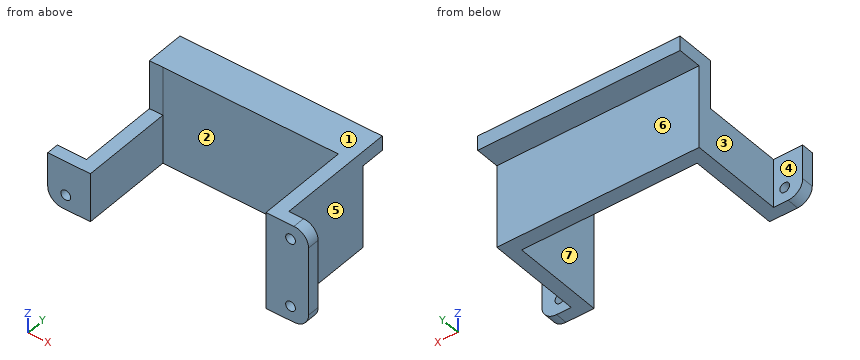
from build123d import *

# Parameters (mm, degrees)
BOSS_EXTRUDE1_DEPTH      = 33.5
SKETCH2_W                = 20
SKETCH2_H                = 2.5
BOSS_EXTRUDE2_DEPTH      = 6
SKETCH9_R                = 1
CORTE_EXTRUS_O1_DEPTH    = 48.67140128
FILETE1_R                = 3
ESBO_O12_W               = 41.5
ESBO_O12_H               = 3
RESSALTO_EXTRUS_O1_DEPTH = 5
FILETE1_OF_ESPELHAR1_R   = 3
ESBO_O14_W               = 12
ESBO_O14_H               = 19.002666305
CORTE_EXTRUS_O10_DEPTH   = 10
ESBO_O15_W               = 13.5
ESBO_O15_H               = 22.081303671
CORTE_EXTRUS_O11_DEPTH   = 62.469504634


with BuildPart() as part:
    # Sketch1 → Boss-Extrude1 (new body)
    with BuildSketch(Plane.XY):
        Polygon((19, -20), (21.75, -20), (21.75, 2), (-19.75, 2), (-19.75, -20), (-17, -20), (-17, -1), (19, -1), align=None)
    extrude(amount=BOSS_EXTRUDE1_DEPTH)

    # Sketch2 → Boss-Extrude2 (add)
    with BuildSketch(Plane(origin=(21.75, 0, 0), x_dir=(0, 0, -1), z_dir=(1, 0, 0))):
        with Locations((-23.5, -18.75)):
            Rectangle(SKETCH2_W, SKETCH2_H)
    boss_extrude2 = extrude(amount=BOSS_EXTRUDE2_DEPTH)

    # Sketch9 → Corte-extrusão1 (cut, through all)
    with BuildSketch(Plane(origin=(0, -17.5, 0), x_dir=(1, 0, 0), z_dir=(0, 1, 0))):
        with Locations(Location((24.05, -16.5, 0), (0, 0, 270))):
            Circle(SKETCH9_R)
        with Locations(Location((24.05, -30.5, 0), (0, 0, 270))):
            Circle(SKETCH9_R)
    corte_extrus_o1 = extrude(amount=-CORTE_EXTRUS_O1_DEPTH, mode=Mode.SUBTRACT)

    # Filete1
    filete1_edges = [part.edges().sort_by_distance(p)[0] for p in [
        (27.75, -18.75, 13.5),
        (27.75, -18.75, 33.5),
    ]]
    fillet(filete1_edges, radius=FILETE1_R)

    # Esboço12 → Ressalto-extrusão1 (add)
    with BuildSketch(Plane(origin=(0, 2, 0), x_dir=(1, 0, 0), z_dir=(0, 1, 0))):
        with Locations((1, -32)):
            Rectangle(ESBO_O12_W, ESBO_O12_H)
    extrude(amount=RESSALTO_EXTRUS_O1_DEPTH)

    # Espelhar1: Boss-Extrude2, Corte-extrusão1 across plane
    add(boss_extrude2.mirror(Plane(origin=(1, 0, 0), x_dir=(0, 0, 1), z_dir=(1, 0, 0))))
    add(corte_extrus_o1.mirror(Plane(origin=(1, 0, 0), x_dir=(0, 0, 1), z_dir=(1, 0, 0))), mode=Mode.SUBTRACT)

    # Filete1 of Espelhar1
    filete1_of_espelhar1_edges = [part.edges().sort_by_distance(p)[0] for p in [
        (-25.75, -18.75, 13.5),
        (-25.75, -18.75, 33.5),
    ]]
    fillet(filete1_of_espelhar1_edges, radius=FILETE1_OF_ESPELHAR1_R)

    # Esboço14 → Corte-extrusão10 (cut)
    with BuildSketch(Plane.XY.offset(33.5)):
        with Locations((-23, -10.498666848)):
            Rectangle(ESBO_O14_W, ESBO_O14_H)
    extrude(amount=-CORTE_EXTRUS_O10_DEPTH, mode=Mode.SUBTRACT)

    # Esboço15 → Corte-extrusão11 (cut, through all)
    with BuildSketch(Plane.ZY.offset(19.75)):
        with Locations((6.75, -8.959348164)):
            Rectangle(ESBO_O15_W, ESBO_O15_H)
    extrude(amount=-CORTE_EXTRUS_O11_DEPTH, mode=Mode.SUBTRACT)


solid = part.part
Check sheet for the modelled part. Datum: model origin and axes. Units: mm. Face numbers are marked on the shaded views. A direction names the side the tool comes from. Give positions to 0.01 mm unless a question says otherwise; leave off trailing zeros. Loops run counter-clockwise (first coordinate to the right, second up) from the corner with the lowest first, then second, coordinate; pieces in that order, holes last. Notation, with made-up numbers: M -10,-13 L 12,-13 A25 cw 12,6 Z; hole C 73,31.5 d6. An arc over 180 degrees is marked long. Answer as a JSON object with one key per item and string values. Group by question number.
Q1. Cross-section at C-C on x = 24.05. Record the cut outline in (y, z).
Q2. Cross-section at A-A on y = -13. Record the cut outline in (x, z).
Q3. Go/stop test with flat-tipped pins: P1, Ø5, axis at x = -23.5, z = 16, coming from the +Y side; P2, Ø6, axis at y = -12, z = 28.5, coming from the +X side; P3, Ø3, axis at x = -18, z = 29, coming from the -Y side. Record where each tip stops, or that it passes through.
Q4. Release check for a two-part mould opening along X. For the marked faces 1, 2 and 3 record: released by +X, released by -X, zero draft, split by the parting line, or undercut.
Q5. Material ranges on line 1 along X through (y, z) = (-18.4, 16.5); line 2 along X through (y, z) = (-16.5, 18); line 3 along Z through (x, y) = (-22.05, -19.5), recorded low to high. Write a range as [from, to].
Q6. Cross-section at B-B on x = -22.05. Record the cut outline in (y, z).
Q7. Access from +Z, -Z, +X, -X, +Y, -Y to the whole of each face (thin tool, end or side, straight path). Record for the marked faces 4, 5, 6 and 7.
Evaluation:
{
 "1": {"outline": "M -20,13.5 L -17.5,13.5 L -17.5,15.5 L -20,15.5 Z; M -20,17.5 L -17.5,17.5 L -17.5,29.5 L -20,29.5 Z; M -20,31.5 L -17.5,31.5 L -17.5,33.5 L -20,33.5 Z"},
 "2": {"outline": "M -19.75,13.5 L -17,13.5 L -17,23.5 L -19.75,23.5 Z; M 19,13.5 L 21.75,13.5 L 21.75,33.5 L 19,33.5 Z"},
 "3": {"P1": "stops at y = -17.5", "P2": "stops at x = 21.75", "P3": "stops at y = -1"},
 "4": {"face 1": "zero draft", "face 2": "undercut", "face 3": "released by -X"},
 "5": {"line 1": "x = [-25.75, -23.05], [-21.05, -17], [19, 23.05], [25.05, 27.75]", "line 2": "x = [-19.75, -17], [19, 21.75]", "line 3": "z = [13.5, 15.5], [17.5, 23.5]"},
 "6": {"outline": "M -20,13.5 L -17.5,13.5 L -17.5,15.5 L -20,15.5 Z; M -20,17.5 L -17.5,17.5 L -17.5,23.5 L -20,23.5 Z"},
 "7": {"face 4": "+Z, -Z, -X, +Y", "face 5": "+Z, -Z, +X, +Y", "face 6": "-Z, +X, -X, +Y", "face 7": "+Z, -Z, -Y"}
}
